```python
from build123d import *

# Parameters (mm, degrees)
SKETCH021_W             = 20
SKETCH021_H             = 24.05
PAD010_DEPTH            = 6.46
POCKET008_DEPTH         = 4.86
SKETCH022_W             = 1.3
SKETCH022_H             = 14.9
PAD011_DEPTH            = 17.65
SKETCH023_W             = 2.9
SKETCH023_H             = 14.9
PAD012_DEPTH            = 1.6
FILLET017_R             = 1
BODY003_PLACEMENT_ANGLE = 90


with BuildPart() as part:
    # Sketch021 → Pad010 (new body)
    with BuildSketch(Plane.XY):
        with Locations((0, 12.025)):
            Rectangle(SKETCH021_W, SKETCH021_H)
    extrude(amount=PAD010_DEPTH)

    # Sketch020 (on Face6 of Pad010) → Pocket008 (cut)
    with BuildSketch(Plane.XY.offset(6.46)):
        Polygon((7.6, 2.65), (7.6, 21.65), (5.2, 24.05), (-5.2, 24.05), (-7.6, 21.65), (-7.6, 2.65), (-6, 2.65), (-6, 0), (6, 0), (6, 2.65), align=None)
    extrude(amount=-POCKET008_DEPTH, mode=Mode.SUBTRACT)

    # Sketch022 → Pad011 (join)
    with BuildSketch(Plane.XY):
        with Locations((-9.35, 7.5)):
            Rectangle(SKETCH022_W, SKETCH022_H)
    pad011 = extrude(amount=PAD011_DEPTH)

    # Sketch023 (on Face23 of Pad011) → Pad012 (join)
    with BuildSketch(Plane.XY.offset(17.65)):
        with Locations((-8.55, 7.5)):
            Rectangle(SKETCH023_W, SKETCH023_H)
    pad012 = extrude(amount=PAD012_DEPTH)

    # Mirrored004: Pad011, Pad012 across Sketch022 V_Axis
    add(pad011.mirror(Plane(origin=(0, 0, 0), x_dir=(0, 0, 1), z_dir=(1, 0, 0))))
    add(pad012.mirror(Plane(origin=(0, 0, 0), x_dir=(0, 0, 1), z_dir=(1, 0, 0))))

    # Fillet017
    fillet017_edges = [part.edges().sort_by_distance(p)[0] for p in [
        (7.1, 7.5, 19.25),
        (-7.1, 7.5, 19.25),
    ]]
    fillet(fillet017_edges, radius=FILLET017_R)


with BuildPart() as part_1:
    # Body003 placement: moved
    add(part.part.moved(Location((-39, 17.65, 5.75))).rotate(Axis((-39, 17.65, 5.75), (1, 0, 0)), BODY003_PLACEMENT_ANGLE))


solid = part_1.part
```
Geometry: final body of the model. Coordinates: model frame, mm. A direction names the side the tool comes from. Round coordinates to 2 decimals unless told otherwise and drop trailing zeros. Loops run counter-clockwise (first coordinate to the right, second up) from the corner with the lowest first, then second, coordinate; pieces in that order, holes last. Notation, with made-up numbers: (49.5, -10.75) -> (98.5, -10.75) arc R26 cw to (98.5, 28.25) -> close; hole circle Ø3 at (8, 4.25). An arc over 180 degrees is marked (long way). Write each question's results on one line, items separated by ' | '.
Item 1: Set-up query: faces 1 (the face through (-31.4, 14, 18)), 2 (the face through (-48, 5, 20.7)), 3 (the face through (-33, 14, 29)), 4 (the face through (-47, 0, 13)), 5 (the face through (-31.615, -1.299, 13.354)). Return all of +Z, -Z, +X, -X, +Y, -Y with unobstructed straight access to the full face (end or side cutting, diameter ignored); none if empty.
Answers below:
face 1: none | face 2: +Z, +X, -X, -Y | face 3: -Y | face 4: +Z, -Z | face 5: +Z, -Z, -Y
Item 2: Cut plane C-C on y = 15. Return the cut outline in (x, z), and give its area (3 significant figures).
Answers below:
outline: (-49, 5.75) -> (-45, 5.75) -> (-45, 8.4) -> (-46.6, 8.4) -> (-46.6, 27.4) -> (-44.2, 29.8) -> (-49, 29.8) -> close; (-33.8, 29.8) -> (-31.4, 27.4) -> (-31.4, 8.4) -> (-33, 8.4) -> (-33, 5.75) -> (-29, 5.75) -> (-29, 29.8) -> close | area: 130 mm²
Item 3: Pull-direction query (Z, two-part tool) for faces 6 (the face through (-39, 16.05, 18)), 7 (the face through (-31, 0, 13)), 8 (the face through (-39, 17, 29.8)); classes: pulls with the +Z half, pulls with the -Z half, needs draft (parallel to the pull), parting line crosses it, or undercut.
Answers below:
face 6: undercut | face 7: needs draft | face 8: pulls with the +Z half
Item 4: Line query: probe 1 along X at (y, z) = (14.25, 12); probe 2 along Y at (x, z) = (-30.75, 15.25); probe 3 along X at (y, z) = (-0.5, 11.75). Output: solid intervals per line, ascending. Write a range as [from, to].
Answers below:
probe 1: x = [-49, -46.6], [-31.4, -29] | probe 2: y = [-1.6, 0], [11.19, 17.65] | probe 3: x = [-49, -46.1], [-31.9, -29]
Item 5: Cut plane D-D on x = -34.5. Return the cut outline in (y, z).
Answers below:
outline: (16.05, 5.75) -> (17.65, 5.75) -> (17.65, 29.8) -> (16.05, 29.8) -> close
Item 6: Cut plane A-A on y = 8.5. Return the cut outline in (x, z).
Answers below:
outline: (-49, 5.8) -> (-47.7, 5.8) -> (-47.7, 20.7) -> (-49, 20.7) -> close; (-30.3, 5.8) -> (-29, 5.8) -> (-29, 20.7) -> (-30.3, 20.7) -> close
Item 7: Cut plane B-B on z = 12.75. Return the cut outline in (x, y), and give its area (3 significant figures).
Answers below:
outline: (-49, -1.6) -> (-47.1, -1.6) arc R1 ccw to (-46.1, -0.6) -> (-46.1, 0) -> (-47.7, 0) -> (-47.7, 11.19) -> (-46.6, 11.19) -> (-46.6, 16.05) -> (-31.4, 16.05) -> (-31.4, 11.19) -> (-30.3, 11.19) -> (-30.3, 0) -> (-31.9, 0) -> (-31.9, -0.6) arc R1 ccw to (-30.9, -1.6) -> (-29, -1.6) -> (-29, 17.65) -> (-49, 17.65) -> close | area: 93.3 mm²
Item 8: Pin query (flat end, axial travel): pin 1 Ø2 at (x, z) = (-45, 21) entering from -Y; pin 2 Ø3 at (x, y) = (-47.5, 6.5) entering from +Z; pin 3 Ø2.5 at (x, y) = (-48, 7) entering from -Z. Return the tip coordinate at first contact, or that it passes through.
Answers below:
pin 1: stops at y = 16.05 | pin 2: stops at z = 20.7 | pin 3: stops at z = 5.8
